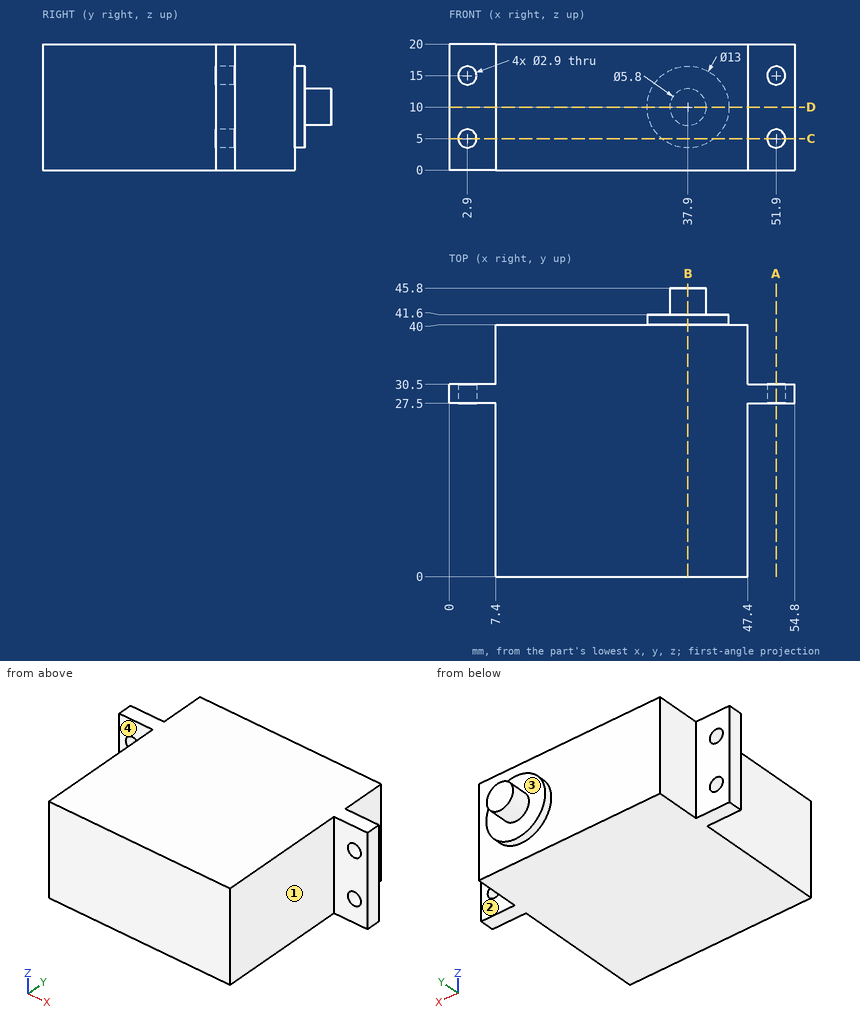
Geometry check sheet. Reference: drawing and pictorial views, mm from the part's lowest x, y, z. A direction names the side the tool comes from. Round coordinates to 2 decimals unless told otherwise and drop trailing zeros. Loops run counter-clockwise (first coordinate to the right, second up) from the corner with the lowest first, then second, coordinate; pieces in that order, holes last. Notation, with made-up numbers: (-15.5, -28.5) -> (-5.5, -28.5) arc R21 ccw to (-5.5, -5.5) -> close; hole circle Ø11 at (89, 64). An arc over 180 degrees is marked (long way). Answer as a JSON object with one key per item and string values. Group by question number.
Item 1: Cross-section at D-D, the plane z = 10. Record the cut outline in (x, y), plus the area to 3 significant figures.
Item 2: Cross-section at A-A, the plane x = 51.9. Record the cut outline in (y, z).
Item 3: Thickness scan on line 1 along X through (y, z) = (28.35, 5); line 2 along Z through (x, y) = (2.9, 28.75); line 3 along X through (y, z) = (32, 12). Record the ranges inside material, lowest first.
Item 4: Depth check by flat-ended pin: pin 1 Ø5 at (y, z) = (19.5, 5) entering from +X; pin 2 Ø1 at (x, z) = (7.5, 5) entering from +Y; pin 3 Ø6 at (x, z) = (3.5, 9.5) entering from -Y; pin 4 Ø10 at (x, z) = (19, 12.5) entering from -Y. Enter the tip coordinate at first touch or a pass-through.
Item 5: Set-up check for the marked faces 1, 2, 3 and 4: record each of +Z, -Z, +X, -X, +Y, -Y from which the full face is reachable in a straight line by a thin tool's end or side.
Item 6: Cross-section at C-C, the plane z = 5. Record the cut outline in (x, y).
Item 7: Cross-section at B-B, the plane x = 37.9. Record the cut outline in (y, z).
Determined:
{
 "1": {"outline": "(0, 27.5) -> (7.4, 27.5) -> (7.4, 0) -> (47.4, 0) -> (47.4, 27.5) -> (54.8, 27.5) -> (54.8, 30.5) -> (47.4, 30.5) -> (47.4, 40) -> (44.4, 40) -> (44.4, 41.6) -> (40.8, 41.6) -> (40.8, 45.8) -> (35, 45.8) -> (35, 41.6) -> (31.4, 41.6) -> (31.4, 40) -> (7.4, 40) -> (7.4, 30.5) -> (0, 30.5) -> close", "area": "1,690 mm²"},
 "2": {"outline": "(27.5, 0) -> (30.5, 0) -> (30.5, 3.55) -> (27.5, 3.55) -> close; (27.5, 6.45) -> (30.5, 6.45) -> (30.5, 13.55) -> (27.5, 13.55) -> close; (27.5, 16.45) -> (30.5, 16.45) -> (30.5, 20) -> (27.5, 20) -> close"},
 "3": {"line 1": "x = 0 to 1.45, 4.35 to 50.45, 53.35 to 54.8", "line 2": "z = 0 to 3.55, 6.45 to 13.55, 16.45 to 20", "line 3": "x = 7.4 to 47.4"},
 "4": {"pin 1": "stops at x = 47.4", "pin 2": "stops at y = 40", "pin 3": "stops at y = 27.5", "pin 4": "stops at y = 0"},
 "5": {"face 1": "+Z, -Z, +X, -Y", "face 2": "+Z, -Z, +X, +Y", "face 3": "+Y", "face 4": "+Z, -Z, -X, -Y"},
 "6": {"outline": "(0, 27.5) -> (1.45, 27.5) -> (1.45, 30.5) -> (0, 30.5) -> close; (4.35, 27.5) -> (7.4, 27.5) -> (7.4, 0) -> (47.4, 0) -> (47.4, 27.5) -> (50.45, 27.5) -> (50.45, 30.5) -> (47.4, 30.5) -> (47.4, 40) -> (42.05, 40) -> (42.05, 41.6) -> (33.75, 41.6) -> (33.75, 40) -> (7.4, 40) -> (7.4, 30.5) -> (4.35, 30.5) -> close; (53.35, 27.5) -> (54.8, 27.5) -> (54.8, 30.5) -> (53.35, 30.5) -> close"},
 "7": {"outline": "(0, 0) -> (40, 0) -> (40, 3.5) -> (41.6, 3.5) -> (41.6, 7.1) -> (45.8, 7.1) -> (45.8, 12.9) -> (41.6, 12.9) -> (41.6, 16.5) -> (40, 16.5) -> (40, 20) -> (0, 20) -> close"}
}
